Work out the finished part from the listing and answer in its coordinate system (mm). Round coordinates to 2 decimals unless told otherwise and drop trailing zeros. Order: outer loops, then holes, each group sorted by start corner. A loop starts at its lowest first (then second) coordinate and runs counter-clockwise, first axis right, second up. Notation, with made-up numbers: (52.25, 81) - (62.25, 81) arc R27 ccw to (62.25, 109) - close; hole circle Ø1 at (22, 43.25). An arc over 180 degrees is marked (long way). Answer in a Markdown table with one row per item.
from build123d import *

# Parameters (mm, degrees)
SKETCH_1_W          = 170
SKETCH_1_H          = 220
EXTRUDE_1_DEPTH     = 3
SKETCH_3_R          = 1.5
CUT_EXTRUDE_1_DEPTH = 279.044960393
SKETCH_4_R          = 1.5
CUT_EXTRUDE_2_DEPTH = 279.044960393
SKETCH_5_W          = 170
SKETCH_5_H          = 10
CUT_EXTRUDE_3_DEPTH = 279.044960393
SKETCH_7_W          = 140
SKETCH_7_H          = 50
SKETCH_7_H_2        = 70
EXTRUDE_2_DEPTH     = 3
FILLET_1_R          = 10


with BuildPart() as part:
    # 草图1 → 凸台-拉伸1 (new body)
    with BuildSketch(Plane(origin=(0, 0, 0), x_dir=(1, 0, 0), z_dir=(0, 1, 0))):
        with Locations((85, 110)):
            Rectangle(SKETCH_1_W, SKETCH_1_H)
    extrude(amount=EXTRUDE_1_DEPTH)

    # 草图3 → 切除-拉伸1 (cut, through all)
    with BuildSketch(Plane(origin=(0, 3, 0), x_dir=(1, 0, 0), z_dir=(0, 1, 0))):
        with Locations(Location((33, 86, 0), (0, 0, 270))):
            Circle(SKETCH_3_R)
        with Locations(Location((33, 166, 0), (0, 0, 270))):
            Circle(SKETCH_3_R)
    extrude(amount=-CUT_EXTRUDE_1_DEPTH, mode=Mode.SUBTRACT)

    # 草图4 → 切除-拉伸2 (cut, through all)
    with BuildSketch(Plane(origin=(0, 3, 0), x_dir=(1, 0, 0), z_dir=(0, 1, 0))):
        with Locations(Location((12, 195, 0), (0, 0, 270))):
            Circle(SKETCH_4_R)
        with Locations(Location((12, 60, 0), (0, 0, 270))):
            Circle(SKETCH_4_R)
    extrude(amount=-CUT_EXTRUDE_2_DEPTH, mode=Mode.SUBTRACT)

    # 草图5 → 切除-拉伸3 (cut, through all)
    with BuildSketch(Plane(origin=(0, 3, 0), x_dir=(1, 0, 0), z_dir=(0, 1, 0))):
        with Locations((85, 5)):
            Rectangle(SKETCH_5_W, SKETCH_5_H)
    extrude(amount=-CUT_EXTRUDE_3_DEPTH, mode=Mode.SUBTRACT)

    # 草图7 → 凸台-拉伸2 (add)
    with BuildSketch(Plane(origin=(0, 3, 0), x_dir=(1, 0, 0), z_dir=(0, 1, 0))):
        with Locations((100, 245)):
            Rectangle(SKETCH_7_W, SKETCH_7_H)
        with Locations((100, -25)):
            Rectangle(SKETCH_7_W, SKETCH_7_H_2)
    extrude(amount=-EXTRUDE_2_DEPTH)

    # 圆角1
    fillet_1_edges = [part.edges().sort_by_distance(p)[0] for p in [
        (0, 1.5, -10),
        (30, 1.5, -270),
        (30, 1.5, -220),
        (170, 1.5, -270),
        (30, 1.5, -10),
        (30, 1.5, 60),
        (170, 1.5, 60),
        (0, 1.5, -220),
    ]]
    fillet(fillet_1_edges, radius=FILLET_1_R)


solid = part.part
1) Find section A-A, the plane y = 1.3. Give the vertices of the cut face in (x, z).
Filled in:
| item | result |
|---|---|
| outline | (0, -210) arc R10 ccw to (10, -220) - (20, -220) arc R10 cw to (30, -230) - (30, -260) arc R10 ccw to (40, -270) - (160, -270) arc R10 ccw to (170, -260) - (170, 50) arc R10 ccw to (160, 60) - (40, 60) arc R10 ccw to (30, 50) - (30, 0) arc R10 cw to (20, -10) - (10, -10) arc R10 ccw to (0, -20) - close; hole circle Ø3 at (12, -195); hole circle Ø3 at (12, -60); hole circle Ø3 at (33, -166); hole circle Ø3 at (33, -86) |
2) Find section C-C, the plane x = 24. Give the vertices of the cut face in (y, z).
Filled in:
| item | result |
|---|---|
| outline | (0, -220.83) - (3, -220.83) - (3, -9.17) - (0, -9.17) - close |
3) Each of these flat-tipped pins is pushed along its axis until it touches: pin 1 (1.8 mm diameter, centred on x = 33, z = -166, fed in from -Y) (3 decimals); pin 2 (1.5 mm diameter, centred on y = 2, z = 27.5, fed in from -X); pin 3 (0.9 mm diameter, centred on x = 16.5, y = 1, fed in from -Z). Where does it stop, or does it pass through?
Filled in:
| item | result |
|---|---|
| pin 1 | passes through |
| pin 2 | stops at x = 30 |
| pin 3 | stops at z = -220 |
4) Find the intervals of material crossed by probe 1 along X at (y, z) = (1.4, -195); probe 2 along Z at (x, y) = (11.5, 1.5); probe 3 along X at (y, z) = (2.55, 3), in increasing order. Write a range as from..to.
Filled in:
| item | result |
|---|---|
| probe 1 | x = 0..10.5, 13.5..170 |
| probe 2 | z = -220..-196.41, -193.59..-61.41, -58.59..-10 |
| probe 3 | x = 30..170 |
5) Find section B-B, the plane z = -245. Give the vertices of the cut face in (x, y), then the cut area to 3 significant figures.
Filled in:
| item | result |
|---|---|
| outline | (30, 0) - (170, 0) - (170, 3) - (30, 3) - close |
| area | 420 mm^2 |
